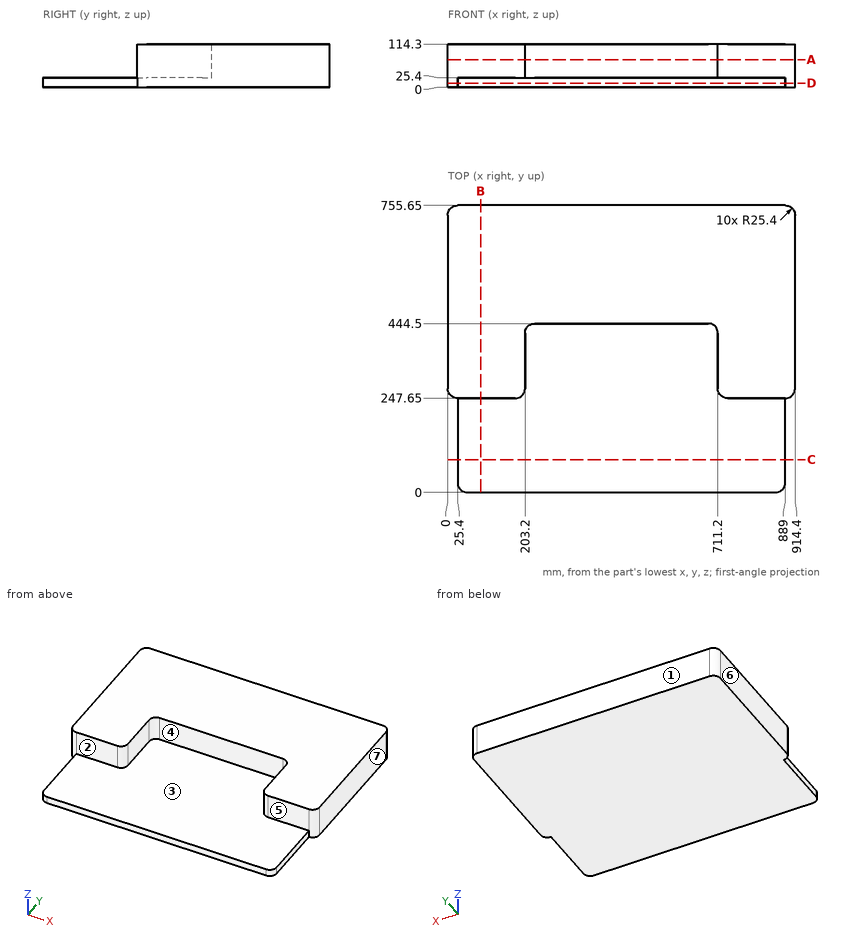
Can you work these out from the drawing? Everything is in mm from the part's minimum corner. A direction names the side the tool comes from. Give positions to 0.01 mm unless a question says otherwise; leave off trailing zeros. Loops run counter-clockwise (first coordinate to the right, second up) from the corner with the lowest first, then second, coordinate; pieces in that order, holes last. Notation, with made-up numbers: (15.5, 29) - (69.5, 29) arc R25 cw to (69.5, 51) - close; hole circle Ø5 at (55, -39.75). An arc over 180 degrees is marked (long way). Answer as a JSON object with one key per item and string values.
Q1. If I drill on L1, parallel to X at y = 358, z = 95; L2, parallel to X at y = 44, z = 6.5; L3, parallel to Y at x = 751.5, z = 38, over which ranges is the centre line in solid material (lowest first)?
Geometry says:
{"L1": "0 to 203.2, 711.2 to 914.4", "L2": "25.4 to 889", "L3": "247.65 to 755.65"}
Q2. Imagine slicing it at B-B on x = 86. Write out the boundary of the cut face in (y, z), plus the area to 3 significant figures.
Geometry says:
{"outline": "(0, 0) - (755.65, 0) - (755.65, 114.3) - (247.65, 114.3) - (247.65, 25.4) - (0, 25.4) - close", "area": "64,400 mm²"}
Q3. Imagine slicing it at D-D on z = 11.5. Write out the boundary of the cut face in (x, y).
Geometry says:
{"outline": "(0, 273.05) arc R25.4 ccw to (25.4, 247.65) - (25.4, 25.4) arc R25.4 ccw to (50.8, 0) - (863.6, 0) arc R25.4 ccw to (889, 25.4) - (889, 247.65) arc R25.4 ccw to (914.4, 273.05) - (914.4, 730.25) arc R25.4 ccw to (889, 755.65) - (25.4, 755.65) arc R25.4 ccw to (0, 730.25) - close"}
Q4. Which directions (+Z, -Z, +X, -X, +Y, -Y) give clear straight access to the entire face, cutting with the end or side of a thin tool? Please do the marked faces 1, 2 and 3.
Geometry says:
{"face 1": "+Z, -Z, +X, -X, +Y", "face 2": "+Z, +X, -X, -Y", "face 3": "+Z, -Y"}
Q5. Imagine slicing it at A-A on z = 73. Write out the boundary of the cut face in (x, y), plus the area to 3 significant figures.
Geometry says:
{"outline": "(0, 273.05) arc R25.4 ccw to (25.4, 247.65) - (177.8, 247.65) arc R25.4 ccw to (203.2, 273.05) - (203.2, 419.1) arc R25.4 cw to (228.6, 444.5) - (685.8, 444.5) arc R25.4 cw to (711.2, 419.1) - (711.2, 273.05) arc R25.4 ccw to (736.6, 247.65) - (889, 247.65) arc R25.4 ccw to (914.4, 273.05) - (914.4, 730.25) arc R25.4 ccw to (889, 755.65) - (25.4, 755.65) arc R25.4 ccw to (0, 730.25) - close", "area": "364,000 mm²"}
Q6. If we mould it in two halves opening along X, with no side actions, what happens to the marked faces 4, 5, 6 and 7? For each: pulls with the +X half, pulls with the -X half, needs draft (parallel to the pull), parting line crosses it, or undercut.
Geometry says:
{"face 4": "undercut", "face 5": "needs draft", "face 6": "pulls with the -X half", "face 7": "pulls with the +X half"}
Q7. Imagine slicing it at C-C on y = 86. Write out the boundary of the cut face in (x, z), plus the area to 3 significant figures.
Geometry says:
{"outline": "(25.4, 0) - (889, 0) - (889, 25.4) - (25.4, 25.4) - close", "area": "21,900 mm²"}
Q8. Will these pins go through, and if not, where does the flat tip stop? P1, Ø8, axis at x = 539, z = 75, coming from the -Y side; P2, Ø3, axis at y = 204.5, z = 20, coming from the -X side; P3, Ø12, axis at x = 784.5, y = 146, coming from the +Z side.
Geometry says:
{"P1": "y = 444.5", "P2": "x = 25.4", "P3": "z = 25.4"}
